Autodesk Inventor part; units mm, degrees
ref_plane "YZ Plane" through (0, 0, 0) normal (1, 0, 0) x (0, 1, 0)
ref_plane "XZ Plane" through (0, 0, 0) normal (0, 1, 0) x (-1, 0, 0)
ref_plane "XY Plane" through (0, 0, 0) normal (0, 0, 1) x (1, 0, 0)
sketch "Szkic1" plane through (0, 0, 0) normal (0, 0, 1) x (1, 0, 0)
  line L0 (0, 0) -> (20, 0)
  line L1 (0, 0) -> (-20, 0)
  line L2 (-20, 0) -> (-20, 20)
  line L3 (-20, 0) -> (0, 0) construction
  line L4 (-20, 20) -> (20, 20)
  line L5 (20, 20) -> (20, 0)
  line L6 (-20, 0) -> (-20, 88)
  line L7 (-20, 88) -> (20, 88)
  line L8 (20, 88) -> (20, 20)
  line L9 (20, 88) -> (20, 93)
  line L10 (20, 93) -> (-20, 93)
  line L11 (-20, 93) -> (-20, 88)
  line L12 (0, 93) -> (35, 93)
  line L13 (35, 93) -> (40, 93)
  line L14 (0, 93) -> (-35, 93)
  line L15 (-35, 93) -> (-40, 93)
  line L16 (-40, 93) -> (-40, 103)
  line L17 (-40, 103) -> (40, 103)
  line L18 (40, 103) -> (40, 93)
  line L19 (-35, 93) -> (-35, 103)
  line L20 (35, 93) -> (35, 103)
  circle A0 centre (-35, 103) radius 1.5
  circle A1 centre (-35, 93) radius 1.5
  circle A2 centre (35, 103) radius 1.5
  circle A3 centre (35, 93) radius 1.5
  line L21 (40, 93) -> (40, 83)
  line L22 (40, 83) -> (20, 83)
  line L23 (-40, 93) -> (-40, 83)
  line L24 (-40, 83) -> (-20, 83)
  line L25 (-40, 103) -> (-40, 183)
  line L26 (40, 103) -> (40, 183)
  line L27 (40, 183) -> (-40, 183)
  dimension "d0" = 20
  dimension "d1" = 20
  dimension "d2" = 20
  dimension "d3" = 90
  dimension "d4" = 88
  dimension "d5" = 5
  dimension "d6" = 35
  dimension "d7" = 5
  dimension "d8" = 35
  dimension "d9" = 5
  dimension "d10" = 10
  dimension "d11" = 3
  dimension "d12" = 3
  dimension "d13" = 3
  dimension "d14" = 3
  dimension "d15" = 10
  dimension "d16" = 10
  dimension "d17" = 80
  dimension "d18" = 80
extrude "Wyciągnięcie proste1" add sketch "Szkic1" along normal blind 8
sketch "Szkic2" plane through (0, 0, 8) normal (0, 0, 1) x (1, 0, 0)
  circle A0 centre (-35, 103) radius 1.5
  circle A1 centre (-35, 93) radius 1.5
  circle A2 centre (35, 103) radius 1.5
  circle A3 centre (35, 93) radius 1.5
  line L0 (-35, 103) -> (35, 103)
  line L1 (-35, 93) -> (35, 93)
  line L2 (-35, 103) -> (-20, 103)
  line L3 (-20, 103) -> (-20, 93)
  line L4 (35, 103) -> (20, 103)
  line L5 (20, 103) -> (20, 93)
  circle A4 centre (-20, 103) radius 2
  circle A5 centre (-20, 93) radius 2
  circle A6 centre (20, 103) radius 2
  circle A7 centre (20, 93) radius 2
  line L6 (40, 83) -> (40, 183)
  line L7 (40, 183) -> (-40, 183)
  line L8 (-40, 183) -> (-40, 83)
  line L9 (-40, 83) -> (-20, 83)
  line L10 (-20, 83) -> (-20, 0)
  line L11 (-20, 0) -> (20, 0)
  line L12 (20, 0) -> (20, 83)
  line L13 (20, 83) -> (40, 83)
  line L14 (-20, 0) -> (20, 0)
  line L15 (-20, 0) -> (-20, 10)
  line L16 (-20, 83) -> (-20, 0)
  line L17 (-20, 10) -> (20, 10)
  line L18 (-20, 10) -> (-10, 10)
  line L19 (20, 10) -> (10, 10)
  circle A8 centre (-10, 10) radius 3
  circle A9 centre (10, 10) radius 3
  point P0 (0, 0)
  dimension "d21" = 15
  dimension "d22" = 15
  dimension "d23" = 4
  dimension "d24" = 4
  dimension "d25" = 4
  dimension "d26" = 4
  dimension "d27" = 10
  dimension "d28" = 10
  dimension "d29" = 10
  dimension "d30" = 6
  dimension "d31" = 6
hole "Otwór1" at (-20, 103, 8) at (-20, 93, 8) at (20, 103, 8) at (20, 93, 8) at (-35, 103, 8) at (-35, 93, 8) at (35, 103, 8) at (35, 93, 8) direction (0, 0, -1) diameter 4 end through all
sketch "Szkic3" plane through (0, 0, 8) normal (0, 0, 1) x (1, 0, 0)
  circle A0 centre (-10, 10) radius 3
  circle A1 centre (10, 10) radius 3
  point P0 (0, 0)
hole "Otwór2" at (-10, 10, 8) at (10, 10, 8) direction (0, 0, -1) diameter 6 end through all
fillet "Zaokrąglenie1" radius 20 2 edges at (20, 83, 4) (-20, 83, 4)
sketch "Szkic4" plane through (0, 0, 8) normal (0, 0, 1) x (1, 0, 0)
  line L0 (40, 183) -> (-40, 183)
  line L1 (40, 83) -> (40, 183)
  line L2 (40, 183) -> (-40, 183)
  line L3 (-40, 183) -> (-40, 333)
  line L4 (-40, 333) -> (0, 333)
  line L5 (40, 183) -> (40, 233)
  line L6 (40, 233) -> (0, 333)
  point P0 (0, 0)
  dimension "d47" = 150
  dimension "d50" = 50
extrude "Wyciągnięcie proste2" add sketch "Szkic4" against normal up to surface (8 mm away)
sketch "Szkic5" plane through (0, 0, 8) normal (0, 0, 1) x (1, 0, 0)
  line L0 (0, 333) -> (-40, 333)
  line L1 (-40, 333) -> (-40, 83)
  line L2 (-40, 333) -> (-40, 303)
  line L3 (-40, 303) -> (-15, 303)
  circle A0 centre (-15, 303) radius 15
  point P0 (0, 0)
  dimension "d51" = 30
  dimension "d52" = 25
  dimension "d53" = 30
extrude "Wyciągnięcie proste3" cut sketch "Szkic5" against normal up to next
properties part number "Wspornik pionowy osi Y"
Model file for the job. Use its own axes, mm. A direction names the side the tool comes from. Round coordinates to 2 decimals unless told otherwise and drop trailing zeros. Write each loop counter-clockwise with the first axis right and the second up, starting at its lowest first coordinate (ties: lowest second). Pieces come first, ordered by that corner, then holes. Notation, with made-up numbers: (44, 52.5) - (85, 52.5) arc R8 ccw to (85, 66.5) - close; hole circle Ø3 at (-11, 4). An arc over 180 degrees is marked (long way). One line per item, written item: value.
(1) Two-plate mould, pull along Y, no slides. Class faces 1 (the flat face through (-1, 169, 8)), 2 (the cylindrical face through (-16.953, 317.872, 4.056)), 3 (the flat face through (20.28, 282.3, 4.06)), 4 (the cylindrical face through (-8.2, 12.4, 3.9)): pulls with the +Y half, pulls with the -Y half, needs draft (parallel to the pull), parting line crosses it, or undercut.
Values follow:
face 1: needs draft
face 2: undercut
face 3: pulls with the +Y half
face 4: undercut
(2) 3-axis set-ups, long thin cutter, end or side, ignore diameter. For faces 5 (the flat face through (-40, 206, 4)), 6 (the flat face through (20, 32, 4)), 7 (the flat face through (-20, 31, 4)): which of +Z, -Z, +X, -X, +Y, -Y reach the whole face in a straight line?
Values follow:
face 5: +Z, -Z, -X, +Y, -Y
face 6: +Z, -Z, +X, -Y
face 7: +Z, -Z, -X, -Y
(3) Cut at B-B, the plane z = 2.5. Give the number of separate pieces and of enclosed holes in the cut face, plus the area to 3 significant figures.
Values follow:
separate pieces: 1
enclosed holes: 11
area: 20,600 mm²
(4) Cut at C-C, the plane y = 257. Give the cut face in (x, z), plus the area to 3 significant figures.
Values follow:
outline: (-40, 0) - (30.4, 0) - (30.4, 8) - (-40, 8) - close
area: 563 mm²
(5) Cut at A-A, the plane y = 303. Give the cut face in (x, z).
Values follow:
outline: (-40, 0) - (-30, 0) - (-30, 8) - (-40, 8) - close; (0, 0) - (12, 0) - (12, 8) - (0, 8) - close
(6) Wall check: probe 1 along X at (y, z) = (93, 2); probe 2 along Y at (x, z) = (-35, 3.5); probe 3 along Y at (x, z) = (-14, 1.25). Give the ranges that are in metal, low to high.
Values follow:
probe 1: x = -40 to -37, -33 to -22, -18 to 18, 22 to 33, 37 to 40
probe 2: y = 82.37 to 91, 95 to 101, 105 to 333
probe 3: y = 0 to 288.03, 317.97 to 333
